from build123d import *

# Parameters (mm, degrees)
CUT_EXTRUDE1_DEPTH = 2.38125
SKETCH3_OUTSIDE_W  = 57.48
SKETCH3_OUTSIDE_H  = 57.48
CUT_EXTRUDE2_DEPTH = 12.7


with BuildPart() as part:
    # Sketch1 → Revolve1 (revolve)
    with BuildSketch(Plane.XY):
        Polygon((-46.181818182, -7.851196491), (-46.181818182, -1.501196491), (-33.481818182, -1.501196491), (-33.481818182, 0.086303509), (-25.557018182, 0.086303509), (-25.557018182, -1.513896491), (-23.956818182, -1.513896491), (-23.956818182, 0.086303509), (93.518181818, 0.086303509), (93.518181818, 4.848803509), (99.868181818, 4.848803509), (99.868181818, -7.851196491), align=None)
    revolve(axis=Axis((-46.181818182, -7.851196491, 0), (-1, 0, 0)))

    # Sketch2 → Cut-Extrude1 (cut, symmetric)
    with BuildSketch(Plane.XY):
        with BuildLine():
            Line((17.318181818, 5.781363923), (17.318181818, 0.873703509))
            ThreePointArc((17.318181818, 0.873703509), (18.248117788, -1.371360522), (20.493181818, -2.301296491))
            Line((20.493181818, -2.301296491), (49.068181818, -2.301296491))
            ThreePointArc((49.068181818, -2.301296491), (51.313245848, -1.371360522), (52.243181818, 0.873703509))
            Line((52.243181818, 0.873703509), (52.243181818, 5.781363923))
            Line((52.243181818, 5.781363923), (17.318181818, 5.781363923))
        make_face()
    extrude(amount=CUT_EXTRUDE1_DEPTH, both=True, mode=Mode.SUBTRACT)

    # Sketch3 outside → Cut-Extrude2 (cut)
    with BuildSketch(Plane.ZY.offset(46.181818182)):
        with Locations((0, -7.851)):
            Rectangle(SKETCH3_OUTSIDE_W, SKETCH3_OUTSIDE_H)
        Polygon((6.35, -7.851196491), (3.175, -2.351935177), (-3.175, -2.351935177), (-6.35, -7.851196491), (-3.175, -13.350457805), (3.175, -13.350457805), align=None, mode=Mode.SUBTRACT)
    extrude(amount=-CUT_EXTRUDE2_DEPTH, mode=Mode.SUBTRACT)


solid = part.part
Geometry: final body of the model. Coordinates: model frame, mm. A direction names the side the tool comes from. Round coordinates to 2 decimals unless told otherwise and drop trailing zeros. Loops run counter-clockwise (first coordinate to the right, second up) from the corner with the lowest first, then second, coordinate; pieces in that order, holes last.
Q1. Section D-D on x = 3.5. Return loops of the section in (y, z) (1 decimal).
Q2. Section C-C on y = -4. Return loops of the section in (x, z).
Q3. Pull-direction query (Z, two-part tool) for faces 4 (the cylindrical face through (18.5, -1.6, 0)), 5 (the cylindrical face through (96.74, -20.54, -0.56)), 6 (the flat face through (-40, -13.35, 0)); classes: released by +Z, released by -Z, zero draft, split by the parting line, or undercut.
Q4. Pin query (flat end, axial travel): P1, Ø1.5, axis at x = 16, y = -11, coming from the +Z side; P2, Ø1.6, axis at x = 33, y = -2, coming from the -Z side; P3, Ø1.5, axis at y = -4.5, z = -9, coming from the -X side. Return the tip coordinate at first contact, or that it passes through.
Q5. Section B-B on x = 34.5. Return loops of the section in (y, z) (1 decimal).
Q6. Material intervals for L1, parallel to X at y = -5.25, z = -6; L2, parallel to X at y = -19.5, z = 4.5; L3, parallel to Y at x = -37.5, z = -0.5, sorted ascending.
Q7. Access query for faces 1 (the flat face through (-39.92, -5.06, -4.74)), 2 (the flat face through (-39.921, -5.14, 4.785)), 3 (the flat face through (-23.957, -5, 6)). Directions: +Z, -Z, +X, -X, +Y, -Y. A direction counts if a zero-diameter tool reaches every point of the face in a straight line with its end or side. Return the directions, or none.
Evaluation:
1. outline: circle Ø15.9 at (-7.9, 0)
2. outline: (-46.18, -4.13) - (-33.48, -4.13) - (-33.48, -6.94) - (-25.56, -6.94) - (-25.56, -5.03) - (-23.96, -5.03) - (-23.96, -6.94) - (93.52, -6.94) - (93.52, -12.1) - (99.87, -12.1) - (99.87, 12.1) - (93.52, 12.1) - (93.52, 6.94) - (-23.96, 6.94) - (-23.96, 5.03) - (-25.56, 5.03) - (-25.56, 6.94) - (-33.48, 6.94) - (-33.48, 4.13) - (-46.18, 4.13) - close
3. face 4: undercut
3. face 5: split by the parting line
3. face 6: zero draft
4. P1: stops at z = 7.57
4. P2: stops at z = -6.12
4. P3: stops at x = 93.52
5. outline: (-2.3, -2.4) - (-2.3, 2.4) - (-0.3, 2.4) arc R7.9 ccw (long way) to (-0.3, -2.4) - close
6. L1: x = -33.48 to -25.56, -23.96 to 99.87
6. L2: x = 93.52 to 99.87
6. L3: y = -13.35 to -2.35
7. face 1: -Z, -X, +Y
7. face 2: +Z, -X, +Y
7. face 3: none
